from build123d import *

# Parameters (mm, degrees)
F0_W     = 550.4
F0_H     = 268.4
F0_W_2   = 525
F0_H_2   = 243
F1_DEPTH = 79
F2_W     = 47.7
F2_H     = 12.7
F3_DEPTH = 268.4


with BuildPart() as f1:
    # F0 (on Front) → F1 (new body)
    with BuildSketch(Plane.XZ):
        Rectangle(F0_W, F0_H)
        Rectangle(F0_W_2, F0_H_2, mode=Mode.SUBTRACT)
    extrude(amount=-F1_DEPTH)

    # F2 (on face) → F3 (join, through all)
    with BuildSketch(Plane.XY.offset(134.2)):
        with Locations((-251.35, 6.35)):
            Rectangle(F2_W, F2_H)
        with Locations((251.35, 6.35)):
            Rectangle(F2_W, F2_H)
    extrude(amount=-F3_DEPTH)


solid = f1.part
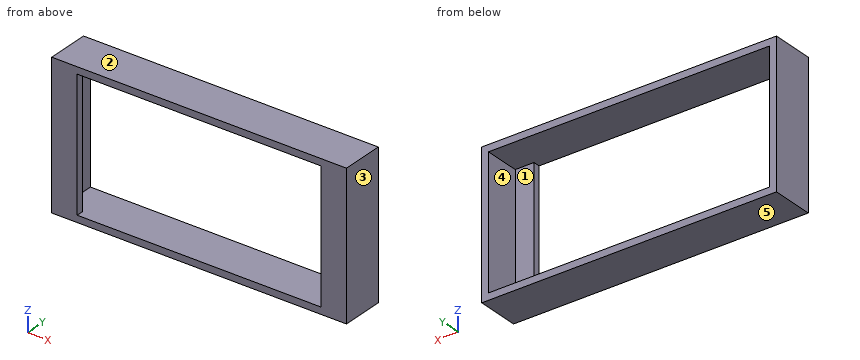
Verification items for the finished model (mm, model axes). Face numbers are marked on the shaded views. A direction names the side the tool comes from. Coordinates: 2 decimals unless noted, no trailing zeros. Order: outer loops, then holes, each group sorted by start corner. A loop starts at its lowest first (then second) coordinate and runs counter-clockwise, first axis right, second up. Notation, with made-up numbers: M 23.5,-9.5 L 82.5,-9.5 A22 ccw 82.5,26.5 Z; hole C 73.25,65.5 d8. An arc over 180 degrees is marked long. Return JSON: item names as keys, results as strings.
1) Cross-section at B-B, the plane z = 14. Record the boundary of the cut face in (x, y).
Answer list:
{"outline": "M -275.2,0 L -227.5,0 L -227.5,12.7 L -262.5,12.7 L -262.5,79 L -275.2,79 Z; M 227.5,0 L 275.2,0 L 275.2,79 L 262.5,79 L 262.5,12.7 L 227.5,12.7 Z"}
2) Cross-section at A-A, the plane x = -151.5. Record the boundary of the cut face in (y, z), and give its area (3 significant figures).
Answer list:
{"outline": "M 0,-134.2 L 79,-134.2 L 79,-121.5 L 0,-121.5 Z; M 0,121.5 L 79,121.5 L 79,134.2 L 0,134.2 Z", "area": "2,010 mm2"}
3) Cross-section at D-D, the plane x = 239. Record the boundary of the cut face in (y, z), and give its area (3 significant figures).
Answer list:
{"outline": "M 0,-134.2 L 79,-134.2 L 79,-121.5 L 12.7,-121.5 L 12.7,121.5 L 79,121.5 L 79,134.2 L 0,134.2 Z", "area": "5,090 mm2"}
4) Gauge pin test, flat end, axial feed: pin 1 (17.5 mm diameter, centred on x = 246, z = 29.5, fed in from +Y). Record the tip position at first contact, or that the pin passes through.
Answer list:
{"pin 1": "y = 12.7"}
5) Thickness scan on L1, parallel to X at y = 62, z = 32; L2, parallel to Z at x = -238.5, y = 44. Record the ranges inside material, lowest first. Write a range as [from, to].
Answer list:
{"L1": "[-275.2, -262.5], [262.5, 275.2]", "L2": "[-134.2, -121.5], [121.5, 134.2]"}
6) Release check for a two-part mould opening along X. For the marked faces 1, 2 and 3 record: +X half, -X half, draft (parallel to the pull), parting line (faces both ways), or undercut.
Answer list:
{"face 1": "undercut", "face 2": "draft", "face 3": "+X half"}
7) Cross-section at C-C, the plane y = 6.5. Record the boundary of the cut face in (x, z).
Answer list:
{"outline": "M -275.2,-134.2 L 275.2,-134.2 L 275.2,134.2 L -275.2,134.2 Z; hole M -227.5,-121.5 L 227.5,-121.5 L 227.5,121.5 L -227.5,121.5 Z"}
8) Access from +Z, -Z, +X, -X, +Y, -Y to the whole of each face (thin tool, end or side, straight path). Record for the marked faces 4 and 5.
Answer list:
{"face 4": "+Y", "face 5": "-Z, +X, -X, +Y, -Y"}
